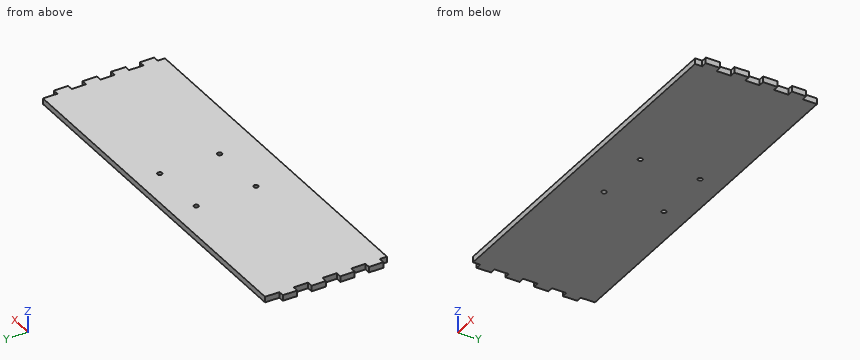
Autodesk Inventor part; units mm, degrees
ref_plane "YZ Plane" through (0, 0, 0) normal (1, 0, 0) x (0, 1, 0)
ref_plane "XZ Plane" through (0, 0, 0) normal (0, 1, 0) x (-1, 0, 0)
ref_plane "XY Plane" through (0, 0, 0) normal (0, 0, 1) x (1, 0, 0)
sketch "Эскиз1" plane through (0, 0, 0) normal (0, 0, 1) x (1, 0, 0)
  line L0 (0, 16.0005) -> (-4, 16.0005)
  line L1 (-4, 6.0005) -> (-4, 16.0005)
  line L2 (-4, 6.0005) -> (0, 6.0005)
  line L3 (0, 16.0005) -> (0, 6.0005)
  line L4 (0, 36.0005) -> (-4, 36.0005)
  line L5 (-4, 26.0005) -> (-4, 36.0005)
  line L6 (-4, 26.0005) -> (0, 26.0005)
  line L7 (0, 36.0005) -> (0, 26.0005)
  line L8 (0, 56.0005) -> (-4, 56.0005)
  line L9 (-4, 46.0005) -> (-4, 56.0005)
  line L10 (-4, 46.0005) -> (0, 46.0005)
  line L11 (0, 56.0005) -> (0, 46.0005)
  line L12 (0, 196.0005) -> (-4, 196.0005)
  line L13 (-4, 186.0005) -> (-4, 196.0005)
  line L14 (-4, 186.0005) -> (0, 186.0005)
  line L15 (0, 196.0005) -> (0, 186.0005)
  line L16 (0, 176.0005) -> (-4, 176.0005)
  line L17 (-4, 166.0005) -> (-4, 176.0005)
  line L18 (-4, 166.0005) -> (0, 166.0005)
  line L19 (0, 176.0005) -> (0, 166.0005)
  line L20 (0, 156.0005) -> (-4, 156.0005)
  line L21 (-4, 146.0005) -> (-4, 156.0005)
  line L22 (-4, 146.0005) -> (0, 146.0005)
  line L23 (0, 156.0005) -> (0, 146.0005)
  line L24 (0, 116.0005) -> (-4, 116.0005)
  line L25 (-4, 106.0005) -> (-4, 116.0005)
  line L26 (-4, 106.0005) -> (0, 106.0005)
  line L27 (0, 116.0005) -> (0, 106.0005)
  line L28 (0, 136.0005) -> (-4, 136.0005)
  line L29 (-4, 126.0005) -> (-4, 136.0005)
  line L30 (-4, 126.0005) -> (0, 126.0005)
  line L31 (0, 136.0005) -> (0, 126.0005)
  line L32 (0, 96.0005) -> (-4, 96.0005)
  line L33 (-4, 86.0005) -> (-4, 96.0005)
  line L34 (-4, 86.0005) -> (0, 86.0005)
  line L35 (0, 96.0005) -> (0, 86.0005)
  line L36 (0, 76.0005) -> (-4, 76.0005)
  line L37 (-4, 66.0005) -> (-4, 76.0005)
  line L38 (-4, 66.0005) -> (0, 66.0005)
  line L39 (0, 76.0005) -> (0, 66.0005)
  line L40 (-194, 0) -> (-194, -4)
  line L41 (-189, -4) -> (-194, -4)
  line L42 (-189, -4) -> (-189, 0)
  line L43 (-194, 0) -> (-189, 0)
  line L44 (-184, 0) -> (-184, -4)
  line L45 (-179, -4) -> (-184, -4)
  line L46 (-179, -4) -> (-179, 0)
  line L47 (-184, 0) -> (-179, 0)
  line L48 (-174, 0) -> (-174, -4)
  line L49 (-169, -4) -> (-174, -4)
  line L50 (-169, -4) -> (-169, 0)
  line L51 (-174, 0) -> (-169, 0)
  line L52 (-164, 0) -> (-164, -4)
  line L53 (-159, -4) -> (-164, -4)
  line L54 (-159, -4) -> (-159, 0)
  line L55 (-164, 0) -> (-159, 0)
  line L56 (-154, 0) -> (-154, -4)
  line L57 (-149, -4) -> (-154, -4)
  line L58 (-149, -4) -> (-149, 0)
  line L59 (-154, 0) -> (-149, 0)
  line L60 (-144, 0) -> (-144, -4)
  line L61 (-139, -4) -> (-144, -4)
  line L62 (-139, -4) -> (-139, 0)
  line L63 (-144, 0) -> (-139, 0)
  line L64 (-14, 0) -> (-14, -4)
  line L65 (-9, -4) -> (-14, -4)
  line L66 (-9, -4) -> (-9, 0)
  line L67 (-14, 0) -> (-9, 0)
  line L68 (-24, 0) -> (-24, -4)
  line L69 (-19, -4) -> (-24, -4)
  line L70 (-19, -4) -> (-19, 0)
  line L71 (-24, 0) -> (-19, 0)
  line L72 (-95.712, 271.7663) -> (-95.712, 277.9752)
  line L73 (-34, 0) -> (-34, -4)
  line L74 (-29, -4) -> (-34, -4)
  line L75 (-29, -4) -> (-29, 0)
  line L76 (-34, 0) -> (-29, 0)
  line L77 (-44, 0) -> (-44, -4)
  line L78 (-39, -4) -> (-44, -4)
  line L79 (-39, -4) -> (-39, 0)
  line L80 (-44, 0) -> (-39, 0)
  line L81 (-54, 0) -> (-54, -4)
  line L82 (-49, -4) -> (-54, -4)
  line L83 (-49, -4) -> (-49, 0)
  line L84 (-54, 0) -> (-49, 0)
  line L85 (-64, 0) -> (-64, -4)
  line L86 (-59, -4) -> (-64, -4)
  line L87 (-59, -4) -> (-59, 0)
  line L88 (-64, 0) -> (-59, 0)
  line L89 (-74, 0) -> (-74, -4)
  line L90 (-69, -4) -> (-74, -4)
  line L91 (-69, -4) -> (-69, 0)
  line L92 (-74, 0) -> (-69, 0)
  line L93 (-84, 0) -> (-84, -4)
  line L94 (-79, -4) -> (-84, -4)
  line L95 (-79, -4) -> (-79, 0)
  line L96 (-84, 0) -> (-79, 0)
  line L97 (-94, 0) -> (-94, -4)
  line L98 (-89, -4) -> (-94, -4)
  line L99 (-89, -4) -> (-89, 0)
  line L100 (-94, 0) -> (-89, 0)
  line L101 (-104, 0) -> (-104, -4)
  line L102 (-99, -4) -> (-104, -4)
  line L103 (-99, -4) -> (-99, 0)
  line L104 (-104, 0) -> (-99, 0)
  line L105 (-114, 0) -> (-114, -4)
  line L106 (-109, -4) -> (-114, -4)
  line L107 (-109, -4) -> (-109, 0)
  line L108 (-114, 0) -> (-109, 0)
  line L109 (-134, 0) -> (-134, -4)
  line L110 (-129, -4) -> (-134, -4)
  line L111 (-129, -4) -> (-129, 0)
  line L112 (-134, 0) -> (-129, 0)
  line L113 (-124, 0) -> (-124, -4)
  line L114 (-119, -4) -> (-124, -4)
  line L115 (-119, -4) -> (-119, 0)
  line L116 (-124, 0) -> (-119, 0)
  line L117 (-263, 126.0005) -> (-263, 136.0005)
  line L118 (-259, 136.0005) -> (-259, 126.0005)
  line L119 (-263, 126.0005) -> (-263, 136.0005)
  line L120 (-259, 136.0005) -> (-259, 126.0005)
  line L121 (-263, 126.0005) -> (-263, 136.0005)
  line L122 (-259, 136.0005) -> (-259, 126.0005)
  line L123 (-263, 126.0005) -> (-263, 136.0005)
  line L124 (-259, 136.0005) -> (-259, 126.0005)
  line L125 (-263, 126.0005) -> (-263, 136.0005)
  line L126 (-259, 136.0005) -> (-259, 126.0005)
  line L127 (-263, 126.0005) -> (-263, 136.0005)
  line L128 (-259, 136.0005) -> (-259, 126.0005)
  line L129 (-259, 136.0005) -> (-263, 136.0005)
  line L130 (-263, 126.0005) -> (-263, 136.0005)
  line L131 (-263, 126.0005) -> (-259, 126.0005)
  line L132 (-259, 136.0005) -> (-259, 126.0005)
  line L133 (-259, 156.0005) -> (-259, 146.0005)
  line L134 (-259, 156.0005) -> (-263, 156.0005)
  line L135 (-263, 146.0005) -> (-263, 156.0005)
  line L136 (-263, 146.0005) -> (-259, 146.0005)
  line L137 (-259, 156.0005) -> (-259, 146.0005)
  line L138 (-259, 176.0005) -> (-263, 176.0005)
  line L139 (-263, 166.0005) -> (-263, 176.0005)
  line L140 (-263, 166.0005) -> (-259, 166.0005)
  line L141 (-259, 176.0005) -> (-259, 166.0005)
  line L142 (-259, 196.0005) -> (-259, 186.0005)
  line L143 (-259, 196.0005) -> (-263, 196.0005)
  line L144 (-263, 186.0005) -> (-263, 196.0005)
  line L145 (-263, 186.0005) -> (-259, 186.0005)
  line L146 (-259, 196.0005) -> (-259, 186.0005)
  line L147 (-4, 196.0005) -> (-4, 206.0005)
  line L148 (-4, 196.0005) -> (0, 196.0005)
  line L149 (0, 206.0005) -> (0, 196.0005)
  line L150 (-4, 206.0005) -> (0, 206.0005)
  line L151 (-263, 196.0005) -> (-263, 206.0005)
  line L152 (-259, 206.0005) -> (-259, 196.0005)
  line L153 (-4, 206.0005) -> (-259, 206.0005)
  line L154 (-259, 206.0005) -> (-259, 0)
  line L155 (-259, 0) -> (-4, 0)
  line L156 (-4, 0) -> (-4, 206.0005)
  line L157 (-204, 0) -> (-204, -4)
  line L158 (-199, -4) -> (-204, -4)
  line L159 (-199, -4) -> (-199, 0)
  line L160 (-204, 0) -> (-199, 0)
  line L161 (-214, 0) -> (-214, -4)
  line L162 (-209, -4) -> (-214, -4)
  line L163 (-209, -4) -> (-209, 0)
  line L164 (-214, 0) -> (-209, 0)
  line L165 (-224, 0) -> (-224, -4)
  line L166 (-219, -4) -> (-224, -4)
  line L167 (-219, -4) -> (-219, 0)
  line L168 (-224, 0) -> (-219, 0)
  line L169 (-234, 0) -> (-234, -4)
  line L170 (-229, -4) -> (-234, -4)
  line L171 (-229, -4) -> (-229, 0)
  line L172 (-234, 0) -> (-229, 0)
  line L173 (-244, 0) -> (-244, -4)
  line L174 (-239, -4) -> (-244, -4)
  line L175 (-239, -4) -> (-239, 0)
  line L176 (-244, 0) -> (-239, 0)
  line L177 (-253.5, 0) -> (-253.5, -4)
  line L178 (-254, 0) -> (-254, -4)
  line L179 (-249, -4) -> (-254, -4)
  line L180 (-249, -4) -> (-249, 0)
  line L181 (-254, 0) -> (-249, 0)
  line L182 (-259, 136.0005) -> (-263, 136.0005)
  line L183 (-263, 126.0005) -> (-259, 126.0005)
  line L184 (-259, 136.0005) -> (-263, 136.0005)
  line L185 (-263, 126.0005) -> (-259, 126.0005)
  line L186 (-259, 136.0005) -> (-263, 136.0005)
  line L187 (-263, 126.0005) -> (-259, 126.0005)
  line L188 (-259, 136.0005) -> (-263, 136.0005)
  line L189 (-263, 126.0005) -> (-259, 126.0005)
  line L190 (-259, 136.0005) -> (-263, 136.0005)
  line L191 (-263, 126.0005) -> (-259, 126.0005)
  line L192 (-259, 136.0005) -> (-263, 136.0005)
  line L193 (-263, 126.0005) -> (-259, 126.0005)
  point P0 (0, 0)
  point P1 (-199, 206.0005)
  point P2 (-259, 176.0005)
  point P3 (-259, 156.0005)
  point P4 (-259, 146.0005)
extrude "Выдавливание1" add sketch "Эскиз1" along normal blind 4 contours L3 L2 L1 L0 | L1 L156 L155 L67 L71 L76 L80 L84 L88 L92 L96 L100 L104 L108 L116 L112 L63 L59 L55 L51 L47 L43 L154 L118 L133 L141 L142 L152 L153 L147 L13 L17 L21 L29 L25 L33 L37 L9 L5 | L5 L4 L7 L6 | L66 L65 L64 L67 | L9 L8 L11 L10 | L70 L69 L68 L71 | L37 L36 L39 L38 | L75 L74 L73 L76 | L33 L32 L35 L34 | L79 L78 L77 L80 | L25 L24 L27 L26 | L83 L82 L81 L84 | L29 L28 L31 L30 | L87 L86 L85 L88 | L21 L20 L23 L22 | L91 L90 L89 L92 | L17 L16 L19 L18 | L95 L94 L93 L96 | L13 L12 L15 L14 | L99 L98 L97 L100 | L103 L102 L101 L104 | L142 L145 L144 L143 | L107 L106 L105 L108 | L141 L140 L139 L138 | L115 L114 L113 L116 | L133 L136 L135 L134 | L111 L110 L109 L112 | L118 L131 L117 L129 | L62 L61 L60 L63 | L155 L177 L179 L178 | L58 L57 L56 L59 | L155 L180 L179 L177 | L54 L53 L52 L55 | L155 L175 L174 L173 | L50 L49 L48 L51 | L155 L171 L170 L169 | L46 L45 L44 L47 | L155 L167 L166 L165 | L42 L41 L40 L43 | L155 L163 L162 L161 | L159 L158 L157 L155
sketch "Эскиз2" plane through (0, 0, 4) normal (0, 0, 1) x (1, 0, 0)
  line L0 (-254, -4) -> (-249, -4)
  line L1 (-254, -4) -> (-263, -4)
  line L2 (-263, 16.0005) -> (-263, 6.0005)
  line L3 (-263, -4) -> (-263, 6.0005)
  line L4 (-263, -4) -> (0, -4)
  line L5 (0, -4) -> (0, 121)
  line L6 (0, 121) -> (-263, 121)
  line L7 (-263, 121) -> (-263, -4)
  point P0 (0, 0)
  dimension "d2" = 125
extrude "Выдавливание2" cut sketch "Эскиз2" against normal blind 10
sketch "Эскиз3" plane through (0, 0, 0) normal (0, 0, -1) x (-1, 0, 0)
  circle A0 centre (110.7056, 189.3601) radius 1.6
  circle A1 centre (152.4249, 189.3601) radius 1.6
  circle A2 centre (152.4249, 147.6408) radius 1.6
  circle A3 centre (110.7056, 147.6408) radius 1.6
  point P0 (0, 0)
extrude "Выдавливание3" cut sketch "Эскиз3" against normal blind 10
properties part number "KB33-046-004-016 - Крышка"
The listing builds one solid part. Answer for the finished solid, in the listing's coordinates (mm). Give positions to 0.01 mm unless a question says otherwise; leave off trailing zeros. Write each loop counter-clockwise with the first axis right and the second up, starting at its lowest first coordinate (ties: lowest second). Pieces come first, ordered by that corner, then holes. Notation, with made-up numbers: (84, 39) -> (142, 39) arc R34 ccw to (142, 76) -> close; hole circle Ø9 at (15, -14.75). An arc over 180 degrees is marked (long way). Use one line per item in the form item = value.
1) Section B-B on z = 1 is taken. Count the separate pieces of the cut face and the enclosed holes in it, plus the area to 3 significant figures.
Result:
separate_pieces = 1
enclosed_holes = 4
area = 22,000 mm²
2) Section A-A on y = 143.5 is taken. Write down the section's boundary in (x, z).
Result:
outline = (-259, 0) -> (-4, 0) -> (-4, 4) -> (-259, 4) -> close
3) Each of these flat-tipped pins is pushed along its axis until it touches: P1, Ø2, axis at x = -1.5, z = 2.5, coming from the -Y side; P2, Ø10, axis at x = -87.5, y = 194.5, coming from the -Z side; P3, Ø2, axis at x = -2, z = 2, coming from the +Y side; P4, Ø2, axis at y = 182.5, z = 1, coming from the +X side. Where does it stop, or does it pass through?
Result:
P1 = 126
P2 = 0
P3 = 196
P4 = -4
4) Straight lines are drawn through the part: probe 1 along X at (y, z) = (149, 3.45); probe 2 along X at (y, z) = (180.5, 3.65). For each, find the intervals that lie inside material, in ascending order.
Result:
probe_1 = -263 to -153.27, -151.58 to -111.55, -109.86 to 0
probe_2 = -259 to -4
